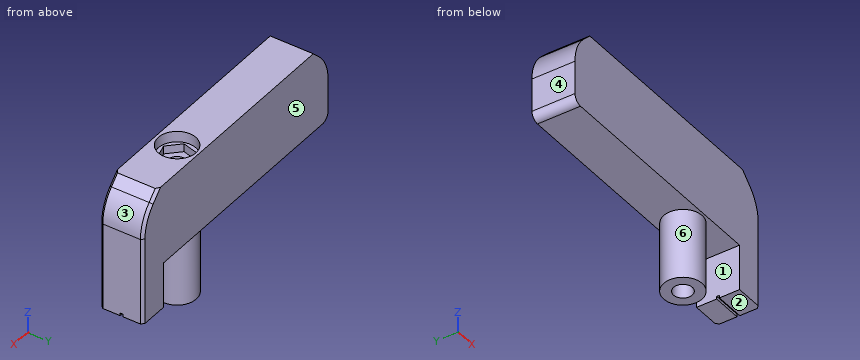
from build123d import *

# Parameters (mm, degrees)
SKETCH_W        = 100
SKETCH_H        = 16
PAD_DEPTH       = 30
SKETCH001_R     = 7.125
PAD001_DEPTH    = 26
SKETCH002_W     = 11
SKETCH002_H     = 16
PAD002_DEPTH    = 17
SKETCH004_R     = 3.5
POCKET_DEPTH    = 56.001
SKETCH005_R     = 7
POCKET001_DEPTH = 4
POCKET002_DEPTH = 7
SKETCH007_W     = 27.137496
SKETCH007_H     = 1
POCKET003_DEPTH = 1
CHAMFER_SIZE    = 8
FILLET_R        = 16
FILLET001_R     = 3
CHAMFER001_SIZE = 1
CHAMFER002_SIZE = 1


with BuildPart() as part:
    # Sketch → Pad (new body)
    with BuildSketch(Plane.XY):
        Rectangle(SKETCH_W, SKETCH_H)
    extrude(amount=PAD_DEPTH)

    # Sketch001 (on Face5 of Pad) → Pad001 (join)
    with BuildSketch(Plane(origin=(0, 0, 0), x_dir=(1, 0, 0), z_dir=(0, 0, -1))):
        with Locations((20, 0)):
            Circle(SKETCH001_R)
    extrude(amount=PAD001_DEPTH)

    # Sketch002 (on Face4 of Pad001) → Pad002 (join)
    with BuildSketch(Plane(origin=(0, 0, 0), x_dir=(1, 0, 0), z_dir=(0, 0, -1))):
        with Locations((44.5, 0)):
            Rectangle(SKETCH002_W, SKETCH002_H)
    extrude(amount=PAD002_DEPTH)

    # Sketch004 (on Face13 of Pad002) → Pocket (cut, through all)
    with BuildSketch(Plane(origin=(0, 0, -26), x_dir=(1, 0, 0), z_dir=(0, 0, -1))):
        with Locations((20, 0)):
            Circle(SKETCH004_R)
    extrude(amount=-POCKET_DEPTH, mode=Mode.SUBTRACT)

    # Sketch005 (on Face6 of Pocket) → Pocket001 (cut)
    with BuildSketch(Plane.XY.offset(30)):
        with Locations((20, 0)):
            Circle(SKETCH005_R)
    extrude(amount=-POCKET001_DEPTH, mode=Mode.SUBTRACT)

    # Sketch006 (on Face6 of Pocket001) → Pocket002 (cut)
    with BuildSketch(Plane.XY.offset(30)):
        Polygon((24.48251, -4.498938), (26.137449, 1.632498), (21.65494, 6.131436), (15.51749, 4.498938), (13.862551, -1.632498), (18.34506, -6.131436), align=None)
    extrude(amount=-POCKET002_DEPTH, mode=Mode.SUBTRACT)

    # Sketch007 (on Face11 of Pocket002) → Pocket003 (cut)
    with BuildSketch(Plane(origin=(0, 0, -17), x_dir=(1, 0, 0), z_dir=(0, 0, -1))):
        with Locations((48.876606, 0)):
            Rectangle(SKETCH007_W, SKETCH007_H)
    extrude(amount=-POCKET003_DEPTH, mode=Mode.SUBTRACT)

    # Chamfer
    chamfer_edges = [part.edges().sort_by_distance(p)[0] for p in [
        (50, 0, 30),
        (-50, 0, 30),
    ]]
    chamfer(chamfer_edges, length=CHAMFER_SIZE)

    # Fillet
    fillet_edges = [part.edges().sort_by_distance(p)[0] for p in [
        (50, 0, 22),
        (-50, 0, 22),
    ]]
    fillet(fillet_edges, radius=FILLET_R)

    # Fillet001
    fillet001_edges = [part.edges().sort_by_distance(p)[0] for p in [
        (-50, 0, 0),
    ]]
    fillet(fillet001_edges, radius=FILLET001_R)

    # Chamfer001
    chamfer001_edges = [part.edges().sort_by_distance(p)[0] for p in [
        (50, 8, -8.5),
    ]]
    chamfer(chamfer001_edges, length=CHAMFER001_SIZE)

    # Chamfer002
    chamfer002_edges = [part.edges().sort_by_distance(p)[0] for p in [
        (50, -8, -8.5),
    ]]
    chamfer(chamfer002_edges, length=CHAMFER002_SIZE)


solid = part.part
Read the model definition and answer for the solid it produces. Units are mm, in the model's axes. Face numbers are marked on the shaded views. A direction names the side the tool comes from. Round coordinates to 2 decimals unless told otherwise and drop trailing zeros. Order: outer loops, then holes, each group sorted by start corner. A loop starts at its lowest first (then second) coordinate and runs counter-clockwise, first axis right, second up.
1) Straight lines are drawn through the part: L1, parallel to X at y = 0, z = -13 (3 decimals); L2, parallel to Y at x = 20, z = 28.1; L3, parallel to Y at x = 20, z = -12 (3 decimals). For each, find the intervals that lie inside material, in ascending order.
2) The mould has two halves that part along X. Classify the marked faces 4, 5 and 6: released by +X, released by -X, zero draft, split by the parting line, or undercut.
3) The part is cut by section C-C on x = 0.5. Write down the section's boundary in (y, z), plus the area to 3 significant figures.
4) For the marked faces 1, 2 and 3, determine the directions among +Z, -Z, +X, -X, +Y, -Y from which every point of the face is accessible in a straight line to the end or side of a thin tool.
5) Flat-ended cylindrical pins translate along their axes: pin 1 (4 mm diameter, centred on x = 43.5, y = 5.5, fed in from -Z); pin 2 (10 mm diameter, centred on x = 5.5, z = -11, fed in from -Y); pin 3 (8 mm diameter, centred on y = -3.5, z = -15, fed in from -X) (3 decimals); pin 4 (1.5 mm diameter, centred on x = -11, y = 5.5, fed in from -Z). Find the tip coordinate at first contact, or state that the pin passes through.
6) The part is cut by section A-A on z = 13.5. Write down the section's boundary in (x, y), plus the area to 3 significant figures.
7) The part is cut by section B-B on x = 20. Write down the section's boundary in (y, z) (3 decimals).
Resolved:
1. L1: x = 12.875 to 16.5, 23.5 to 27.125, 39 to 50
1. L2: y = -8 to -7, 7 to 8
1. L3: y = -7.125 to -3.5, 3.5 to 7.125
2. face 4: released by -X
2. face 5: zero draft
2. face 6: undercut
3. outline: (-8, 0) - (8, 0) - (8, 30) - (-8, 30) - close
3. area: 480 mm2
4. face 1: -Z, +Y, -Y
4. face 2: -Z, +X, +Y, -Y
4. face 3: +Z, +X, +Y, -Y
5. pin 1: stops at z = -17
5. pin 2: passes through
5. pin 3: stops at x = 12.875
5. pin 4: stops at z = 0
6. outline: (-50, -8) - (49, -8) - (50, -7) - (50, 7) - (49, 8) - (-50, 8) - close; hole circle Ø7 at (20, 0)
6. area: 1,560 mm2
7. outline: (-8, 0) - (-7.125, 0) - (-7.125, -26) - (-3.5, -26) - (-3.5, 23) - (-5.691, 23) - (-5.691, 26) - (-7, 26) - (-7, 30) - (-8, 30) - close; (3.5, -26) - (7.125, -26) - (7.125, 0) - (8, 0) - (8, 30) - (7, 30) - (7, 26) - (5.691, 26) - (5.691, 23) - (3.5, 23) - close
